Geometry check sheet. Reference: the model listing, model coordinates, mm. Round coordinates to 2 decimals unless told otherwise and drop trailing zeros. Write each loop counter-clockwise with the first axis right and the second up, starting at its lowest first coordinate (ties: lowest second). Pieces come first, ordered by that corner, then holes.
Item 1: Scan lines: probe 1 along Z at (x, y) = (710, -34.5); probe 2 along Y at (x, z) = (710, 734); probe 3 along Y at (x, z) = (706.25, 384). Record each from-to range of solid material in increasing order.
Item 2: Cross-section at A-A (y = -488). Enter the section's corners in (x, z).
Item 3: Cross-section at D-D (z = 225.5). Enter the section's corners in (x, y), then the cut area to 3 significant figures.
Item 4: Cross-section at C-C (y = -358). Enter the section's corners in (x, z), then the cut area to 3 significant figures.
Item 5: Cross-section at B-B (x = 710). State how many separate pieces and enclosed holes the cut face has, then the cut area to 3 significant figures.
Item 6: Depth check by flat-ended pin: P1, Ø9, axis at x = 710, y = -150, coming from the -Z side; P2, Ø7, axis at y = -150, z = 384, coming from the +X side; P3, Ø4, axis at x = 709, z = 688, coming from the +Y side; P4, Ø6.5, axis at x = 711.5, z = 561.5, coming from the +Y side. Enter the tip coordinate at first touch or a pass-through.
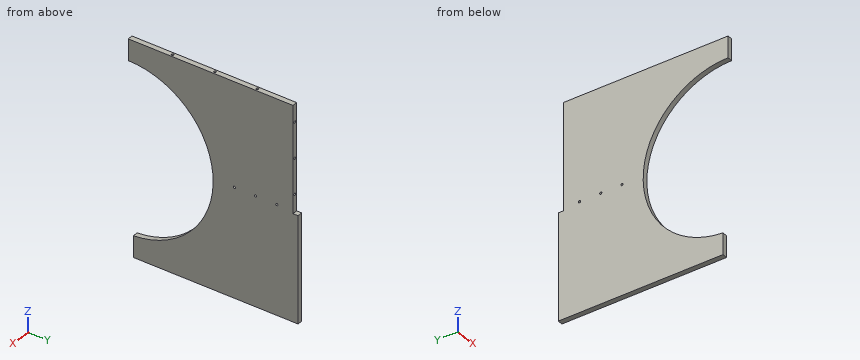
from build123d import *

# Parameters (mm, degrees)
PAD023_DEPTH    = 9
SKETCH069_R     = 4
POCKET020_DEPTH = 30
SKETCH072_R     = 4
POCKET023_DEPTH = 30
SKETCH073_R     = 4
POCKET024_DEPTH = 18.001


with BuildPart() as part:
    # Sketch065 → Pad023 (new body, symmetric)
    with BuildSketch(Plane.YZ):
        with BuildLine():
            Line((-600, 750), (-18, 750))
            Line((-18, 750), (-18, 375))
            Line((-18, 375), (0, 375))
            Line((0, 375), (0, 0))
            Line((0, 0), (-582, 0))
            Line((-582, 0), (-582, 75.270243))
            ThreePointArc((-582, 75.270243), (-300.135152, 383.733813), (-600, 674.729757))
            Line((-600, 750), (-600, 674.729757))
        make_face()
    extrude(amount=PAD023_DEPTH, both=True)

    # Sketch069 (on Face1 of Pad023) → Pocket020 (cut)
    with BuildSketch(Plane(origin=(0, 0, 750), x_dir=(0, -1, 0), z_dir=(0, 0, 1))):
        with Locations((150, 0)):
            Circle(SKETCH069_R)
        with Locations((300, 0)):
            Circle(SKETCH069_R)
        with Locations((450, 0)):
            Circle(SKETCH069_R)
    extrude(amount=-POCKET020_DEPTH, mode=Mode.SUBTRACT)

    # Sketch072 (on Face5 of Pocket020) → Pocket023 (cut)
    with BuildSketch(Plane.ZX.offset(-18)):
        with Locations((437.5, 0)):
            Circle(SKETCH072_R)
        with Locations((562.5, 0)):
            Circle(SKETCH072_R)
        with Locations((687.5, 0)):
            Circle(SKETCH072_R)
    extrude(amount=-POCKET023_DEPTH, mode=Mode.SUBTRACT)

    # Sketch073 (on Face4 of Pocket023) → Pocket024 (cut, through all)
    with BuildSketch(Plane.YZ.offset(9)):
        with Locations((-150, 384)):
            Circle(SKETCH073_R)
        with Locations((-225, 384)):
            Circle(SKETCH073_R)
        with Locations((-75, 384)):
            Circle(SKETCH073_R)
    extrude(amount=-POCKET024_DEPTH, mode=Mode.SUBTRACT)


with BuildPart() as part_1:
    # Body018001001001010001003001003001001019 placement: moved
    add(part.part.moved(Location((-710, 0, 0))))


with BuildPart() as part_2:
    # Clone014 placement: moved
    add(part_1.part.moved(Location((1420, 0, 0))))


solid = part_2.part
Resolved:
1. probe 1: z = 0 to 433.5, 441.5 to 558.5, 566.5 to 683.5, 691.5 to 750
1. probe 2: y = -600 to -454, -446 to -304, -296 to -154, -146 to -18
1. probe 3: y = -300.14 to -229, -221 to -154, -146 to -79, -71 to -18
2. outline: (701, 0) - (719, 0) - (719, 96.42) - (701, 96.42) - close; (701, 653.04) - (719, 653.04) - (719, 750) - (701, 750) - close
3. outline: (701, -339.75) - (719, -339.75) - (719, 0) - (701, 0) - close
3. area: 6,120 mm2
4. outline: (701, 0) - (719, 0) - (719, 197.43) - (701, 197.43) - close; (701, 552.03) - (719, 552.03) - (719, 750) - (701, 750) - close
4. area: 7,120 mm2
5. separate pieces: 1
5. enclosed holes: 3
5. area: 299,000 mm2
6. P1: stops at z = 0
6. P2: passes through
6. P3: stops at y = -48
6. P4: stops at y = -18
